from build123d import *

# Parameters (mm, degrees)
SKETCH1_R                 = 13.97
BOSS_EXTRUDE1_DEPTH       = 87.63
FILLET3_R                 = 2.794
M6X1_0_TAPPED_HOLE1_D     = 5
M6X1_0_TAPPED_HOLE1_DEPTH = 41.148
M6X1_0_TAPPED_HOLE1_TIP   = 1.502151548


with BuildPart() as part:
    # Sketch1 → Boss-Extrude1 (new body)
    with BuildSketch(Plane.XY):
        with BuildLine():
            Line((0, 19.05), (74.609999878, 19.05))
            Line((74.609999878, 19.05), (74.609999878, -19.05))
            Line((74.609999878, -19.05), (0, -19.05))
            ThreePointArc((0, -19.05), (-19.05, 0), (0, 19.05))
        make_face()
        Circle(SKETCH1_R, mode=Mode.SUBTRACT)
    extrude(amount=BOSS_EXTRUDE1_DEPTH)

    # Fillet3
    fillet3_edges = [part.edges().sort_by_distance(p)[0] for p in [
        (-13.97, 0, 0),
    ]]
    fillet(fillet3_edges, radius=FILLET3_R)

    # M6x1.0 Tapped Hole1
    with Locations(Plane(origin=(74.609999878, 0, 0), x_dir=(0, 0, -1), z_dir=(1, 0, 0))):
        with Locations((-80.645, -10.16), (-80.645, 10.16), (-6.985, 10.16), (-6.985, -10.16)):
            Hole(M6X1_0_TAPPED_HOLE1_D / 2, depth=M6X1_0_TAPPED_HOLE1_DEPTH)
            with Locations((0, 0, -(M6X1_0_TAPPED_HOLE1_DEPTH + M6X1_0_TAPPED_HOLE1_TIP / 2))):  # 118° drill point
                Cone(0, M6X1_0_TAPPED_HOLE1_D / 2, M6X1_0_TAPPED_HOLE1_TIP, mode=Mode.SUBTRACT)


solid = part.part
Verification items for the finished model (mm, model axes). A direction names the side the tool comes from. Coordinates: 2 decimals unless noted, no trailing zeros. Loops run counter-clockwise (first coordinate to the right, second up) from the corner with the lowest first, then second, coordinate; pieces in that order, holes last. Notation, with made-up numbers: (-38.5, 81) -> (-2.5, 81) arc R31 ccw to (-2.5, 111) -> close; hole circle Ø1 at (-8.75, -17.5). An arc over 180 degrees is marked (long way). Write each question's results on one line, items separated by ' | '.
Item 1: Section check C-C, the plane z = 23.5. Enter the section's corners in (x, y).
Found:
outline: (0, -19.05) -> (74.61, -19.05) -> (74.61, 19.05) -> (0, 19.05) arc R19.05 ccw to start; hole circle Ø27.94 at (0, 0)
Item 2: Section check A-A, the plane y = 0. Enter the section's corners in (x, z).
Found:
outline: (-19.05, 0) -> (-16.76, 0) arc R2.79 ccw to (-13.97, 2.79) -> (-13.97, 87.63) -> (-19.05, 87.63) -> close; (13.97, 2.79) arc R2.79 ccw to (16.76, 0) -> (74.61, 0) -> (74.61, 87.63) -> (13.97, 87.63) -> close
Item 3: Tool access check on faces 1 (the face through (37, 19.05, 43)), 2 (the face through (53.7, -11.1, 9.3)). Record the directions out of +Z, -Z, +X, -X, +Y, -Y that give a thin tool (end or side, any length) a straight path to the whole face; none if there is none.
Found:
face 1: +Z, -Z, +X, -X, +Y | face 2: +X
Item 4: Gauge pin test, flat ends, axial feed: pin 1 (4 mm diameter, centred on y = 1, z = 60.5, fed in from -X); pin 2 (4.5 mm diameter, centred on y = 10.16, z = 6.985, fed in from -X); pin 3 (4 mm diameter, centred on y = -10.16, z = 80.645, fed in from -X). Record the tip position at first contact, or that the pin passes through.
Found:
pin 1: stops at x = -19.05 | pin 2: stops at x = -17.33 | pin 3: stops at x = -17.21
Item 5: Material ranges on L1, parallel to Z at x = 59, y = 10.16 (3 decimals); L2, parallel to Z at x = 60, y = -10; L3, parallel to Y at x = 55.5, z = 82.5, recorded low to high.
Found:
L1: z = 0 to 4.485, 9.485 to 78.145, 83.145 to 87.63 | L2: z = 0 to 4.49, 9.48 to 78.15, 83.14 to 87.63 | L3: y = -19.05 to -11.84, -8.48 to 8.48, 11.84 to 19.05
Item 6: Section check B-B, the plane x = 60. Enter the section's corners in (y, z) (3 decimals).
Found:
outline: (-19.05, 0) -> (19.05, 0) -> (19.05, 87.63) -> (-19.05, 87.63) -> close; hole circle Ø5 at (-10.16, 6.985); hole circle Ø5 at (-10.16, 80.645); hole circle Ø5 at (10.16, 6.985); hole circle Ø5 at (10.16, 80.645)
Item 7: Mould release check, pull along Z, two halves, no side actions. Record for faces 3 (the face through (74.61, 0, 43)), 4 (the face through (32.22, -10.14, 81.08)), 5 (the face through (39, 0, 87.63)), 6 (the face through (53.748, 9.202, 9.294)): +Z half, -Z half, draft (parallel to the pull), parting line (faces both ways), or undercut.
Found:
face 3: draft | face 4: undercut | face 5: +Z half | face 6: undercut
